Can you work these out from the model? Positions are in its coordinate system, mm. A direction names the side the tool comes from. Give positions to 0.01 mm unless a question says otherwise; leave off trailing zeros. Write each loop counter-clockwise with the first axis right and the second up, starting at its lowest first coordinate (ties: lowest second). Pieces come first, ordered by that corner, then holes. Notation, with made-up numbers: M 80.25,-13 L 95.25,-13 A22 ccw 95.25,20 Z; hole C 70.25,46 d7. An arc over 180 degrees is marked long. Answer as CSV lines item,"result". Start each with the question number.
Autodesk Inventor part; units mm, degrees
ref_plane "YZ Plane" through (0, 0, 0) normal (1, 0, 0) x (0, 1, 0)
ref_plane "XZ Plane" through (0, 0, 0) normal (0, 1, 0) x (-1, 0, 0)
ref_plane "XY Plane" through (0, 0, 0) normal (0, 0, 1) x (1, 0, 0)
sketch "スケッチ1" plane through (0, 0, 0) normal (0, 0, 1) x (1, 0, 0)
  circle A0 centre (-1.476, 8.3709) radius 1.35
  circle A1 centre (0, 0) radius 5.05
  line L0 (-30, 6) -> (-27.5, 6) construction
  line L1 (-27.5, 6) -> (-27.5, -6) construction
  line L2 (-27.5, -6) -> (-30, -6) construction
  line L3 (-30, -6) -> (-30, 6) construction
  line L4 (-27.45, 6.05) -> (-30.05, 6.05) construction
  line L5 (-30.05, 6.05) -> (-30.05, -6.05) construction
  line L6 (-30.05, -6.05) -> (-27.45, -6.05) construction
  line L7 (-27.45, -6.05) -> (-27.45, 6.05) construction
  circle A2 centre (-30.05, 5) radius 1.05 construction
  line L8 (-27.45, 6.05) -> (-30.05, 6.05)
  arc A3 (-30.05, 6.05) -> (-30.05, 3.95) centre (-30.05, 5) ccw
  line L9 (-30.05, 3.95) -> (-30.05, -3.95)
  line L10 (-28.75, 6.05) -> (-28.75, -6.05) construction
  line L11 (-30.05, 0) -> (-27.5, 0) construction
  arc A4 (-30.05, -3.95) -> (-30.05, -6.05) centre (-30.05, -5) ccw
  line L12 (-30.05, -6.05) -> (-27.45, -6.05)
  line L13 (-27.45, 3.95) -> (-27.45, -3.95)
  arc A5 (-27.45, 3.95) -> (-27.45, 6.05) centre (-27.45, 5) ccw
  arc A6 (-27.45, -6.05) -> (-27.45, -3.95) centre (-27.45, -5) ccw
  circle A7 centre (-30, 12) radius 1.55
  circle A8 centre (-30, -12) radius 1.55
  line L14 (-32.5, 16) -> (-27.5, 16)
  line L15 (-32.5, -16) -> (-27.5, -16)
  arc A9 (1.9894, -10.3098) -> (1.9894, 10.3098) centre (0, 0) ccw
  line L16 (-32.5, 16) -> (-32.5, -16)
  line L17 (-27.5, 16) -> (1.9894, 10.3098)
  line L18 (1.9894, -10.3098) -> (-27.5, -16)
  line L19 (-1.476, 8.3709) -> (0, 0) construction
  line L20 (0, 10.6937) -> (0, -10.6937) construction
  circle A10 centre (-8.3709, -1.476) radius 1.35
  circle A11 centre (1.476, -8.3709) radius 1.35
  circle A12 centre (8.3709, 1.476) radius 1.35
  point P0 (-28.775, 0)
  dimension "d29" = 2.1
  dimension "d4" = 2.7
  dimension "d9" = 10.1
  dimension "d10" = 2.5
  dimension "d30" = 0.05
  dimension "d31" = 6
  dimension "d33" = 3.1
  dimension "d57" = 32
  dimension "d61" = 32.5
  dimension "d62" = 5
  dimension "d63" = 2.5
  dimension "d65" = 10
  dimension "d66" = 10.5
  dimension "d67" = 8.5
  dimension "d69" = 10
  dimension "d72" = 360
extrude "押し出し1" add sketch "スケッチ1" along normal blind 2
equation "\"d23\" = 7"
properties part number "Shoulder_side_frame" material "アルミニウム 2014-T4"
1) I want a section at D-D, the plane x = -10.5. Please give me the cut outline in (y, z).
2) I want a section at B-B, the plane z = 0.9. State how many separate pieces and enclosed holes the cut face has, then the cut area to 3 significant figures.
3) I need wall thicknesses on L1, parallel to Y at x = -30, z = 1.25; L2, parallel to Y at x = -1, z = 1.1; L3, parallel to X at y = 2.5, z = 1.7. Which ranges of each line are inside material? Lowest first, please. Write a range as from..to.
4) I want a section at A-A, the plane y = -12. Please give me the cut outline in (x, z).
5) I want a section at C-C, the plane x = 1. Please give me the cut outline in (y, z), then the cut area to 3 significant figures.
6) On a 3-axis mill with a long thin cutter (end or side, diameter ignored), from which of +Z, -Z, +X, -X, +Y, -Y can I reach the whole of each face in a straight line? I mean faces 4 (the cylindrical face through (-31.1, 5, 1)), 5 (the flat face through (-30, -16, 1)). Say none if no direction works.
7) Thinking about a two-plate mould opening in Y: for faces 1 (the flat face through (-16, 0, 2)), 2 (the cylindrical face through (10.5, 0.2, 1)), 3 (the cylindrical face through (1.183, -7.053, 0.986)), which applies, released by +Y, released by -Y, zero draft, split by the parting line, or undercut?
Values found:
1,outline,"M -12.72,0 L 12.72,0 L 12.72,2 L -12.72,2 Z"
2,separate pieces,"1"
2,enclosed holes,"8"
2,area,"911 mm²"
3,L1,"y = -16..-13.55, -10.45..-6.05, 6.05..10.45, 13.55..16"
3,L2,"y = -10.89..-4.95, 4.95..7.11, 9.63..10.89"
3,L3,"x = -32.5..-30.05, -27.45..-4.39, 4.39..7.49, 9.25..10.2"
4,outline,"M -32.5,0 L -31.55,0 L -31.55,2 L -32.5,2 Z; M -28.45,0 L -6.77,0 L -6.77,2 L -28.45,2 Z"
5,outline,"M -10.5,0 L -9.63,0 L -9.63,2 L -10.5,2 Z; M -7.11,0 L -4.95,0 L -4.95,2 L -7.11,2 Z; M 4.95,0 L 10.5,0 L 10.5,2 L 4.95,2 Z"
5,area,"17.1 mm²"
6,face 4,"+Z, -Z"
6,face 5,"+Z, -Z, +X, -X, -Y"
7,face 1,"zero draft"
7,face 2,"split by the parting line"
7,face 3,"undercut"
